from build123d import *

# Parameters (mm, degrees)
SKETCH1_W           = 3.048
SKETCH1_H           = 6.35
BOSS_EXTRUDE1_DEPTH = 3.048


with BuildPart() as part:
    # Sketch1 → Boss-Extrude1 (new body)
    with BuildSketch(Plane.XY):
        Polygon((0, 0), (0, 12.7), (-3.048, 12.7), (-3.048, 25.4), (0, 25.4), (0, 38.1), (-3.048, 38.1), (-3.048, 50.8), (0, 50.8), (0, 63.5), (-3.048, 63.5), (-3.048, 76.2), (6.35, 76.2), (6.35, 82.1944), (12.7, 82.1944), (12.7, 76.2), (19.05, 76.2), (19.05, 82.1944), (25.4, 82.1944), (25.4, 63.5), (28.448, 63.5), (28.448, 50.8), (25.4, 50.8), (25.4, 38.1), (28.448, 38.1), (28.448, 25.4), (25.4, 25.4), (25.4, 12.7), (28.448, 12.7), (28.448, 0), (15.875, 0), (15.875, -5.9944), (9.525, -5.9944), (9.525, 0), align=None)
        with Locations((12.7, 31.75)):
            Rectangle(SKETCH1_W, SKETCH1_H, mode=Mode.SUBTRACT)
    extrude(amount=BOSS_EXTRUDE1_DEPTH)


solid = part.part
Verification items for the finished model (mm, model axes). A direction names the side the tool comes from. Give positions to 0.01 mm unless a question says otherwise; leave off trailing zeros. Write each loop counter-clockwise with the first axis right and the second up, starting at its lowest first coordinate (ties: lowest second). Pieces come first, ordered by that corner, then holes. Notation, with made-up numbers: M 52,88.5 L 87,88.5 A15 ccw 87,113.5 Z; hole C 27.5,-32.75 d9. An arc over 180 degrees is marked long. Use CSV: the item, a comma, the result in double quotes.
1) Release check for a two-part mould opening along X. For faces 5 (the face through (16, 76.2, 2)), 6 (the face through (-3.048, 44, 2)), 7 (the face through (13, 34.925, 2)), 8 (the face through (15.875, -3, 2)) record: released by +X, released by -X, zero draft, split by the parting line, or undercut.
Final values:
face 5,"undercut"
face 6,"released by -X"
face 7,"undercut"
face 8,"released by +X"
2) Material ranges on line 1 along Y through (x, z) = (25.5, 1.05); line 2 along Y through (x, z) = (-1, 1.9); line 3 along X through (y, z) = (30.5, 0.95), recorded low to high.
Final values:
line 1,"0 to 12.7, 25.4 to 38.1, 50.8 to 63.5"
line 2,"12.7 to 25.4, 38.1 to 50.8, 63.5 to 76.2"
line 3,"0 to 11.18, 14.22 to 28.45"
3) Cross-section at B-B (y = 52). Enter the section's corners in (x, z).
Final values:
outline,"M 0,0 L 28.45,0 L 28.45,3.05 L 0,3.05 Z"
4) Access from +Z, -Z, +X, -X, +Y, -Y to the whole of each face (thin tool, end or side, straight path). Record for faces 1 (the face through (6.35, 79, 2)), 2 (the face through (27, 25.4, 2)), 3 (the face through (14.224, 32, 2)), 4 (the face through (-2, 25.4, 2)).
Final values:
face 1,"+Z, -Z, -X, +Y"
face 2,"+Z, -Z, +X"
face 3,"+Z, -Z"
face 4,"+Z, -Z, -X"
5) Cross-section at A-A (x = 24.5). Enter the section's corners in (y, z), plus the area to 3 significant figures.
Final values:
outline,"M 0,0 L 82.19,0 L 82.19,3.05 L 0,3.05 Z"
area,"251 mm²"
6) Go/stop test with flat-tipped pins: pin 1 Ø1.5 at (y, z) = (43.5, 1) entering from +X; pin 2 Ø1.5 at (y, z) = (33, 1) entering from -X. Record where each tip stops, or that it passes through.
Final values:
pin 1,"x = 25.4"
pin 2,"x = 0"
